Could you check a few things on this model? Use its own coordinates, in mm. Coordinates: 2 decimals unless noted, no trailing zeros. Order: outer loops, then holes, each group sorted by start corner. A loop starts at its lowest first (then second) coordinate and runs counter-clockwise, first axis right, second up. Notation, with made-up numbers: (70, -21.75) -> (102, -21.75) arc R28 ccw to (102, 3.25) -> close; hole circle Ø4 at (6, -34). An arc over 180 degrees is marked (long way). Use a Markdown table: item, result. Add a question column.
1) If we section it at B-B (z = 0): Write out the boundary of the cut face in (x, y), plus the area to 3 significant figures.
2) Thinking about a two-plate mould opening in Z: for faces 1 (the flat face through (6.14, -9, -1)), 2 (the cylindrical face through (-6.106, -11.628, -0.256)), 3 (the cylindrical face through (-16.35, -5.74, -0.07)), which applies, +Z half, -Z half, draft (parallel to the pull), parting line (faces both ways), or undercut?
3) If I drill on L1, parallel to X at y = -9, z = 0; L2, parallel to X at y = -3, z = 0; L3, parallel to Z at x = -14.7, y = -2.5, over which ranges is the centre line in solid material (lowest first)? Write a range as [from, to].
4) If we section it at A-A (y = -2.75): Write out the boundary of the cut face in (x, z), plus the area to 3 significant figures.
5) If we section it at D-D (x = 0): Write out the boundary of the cut face in (y, z).
6) Will these pins go through, and if not, where does the flat tip stop? pin 1 Ø5 at (x, z) = (-15.5, 6) entering from -Y; pin 2 Ø12 at (x, z) = (1, 0.5) entering from +Y; pin 3 Ø4 at (x, y) = (-4, -7) entering from -Z.
7) If we section it at C-C (x = -14.7): Write out the boundary of the cut face in (y, z), plus the area to 3 significant figures.
```python
from build123d import *

# Parameters (mm, degrees)
CORTAR_EXTRUIR5_DEPTH = 50
CROQUIS8_R            = 1.65
CORTAR_EXTRUIR6_DEPTH = 50


with BuildPart() as part:
    # Croquis1 → Revolución4 (revolve)
    with BuildSketch(Plane(origin=(0, 0, 0), x_dir=(1, 0, 0), z_dir=(0, 1, 0))):
        with BuildLine():
            Line((-10.7, 0), (-18.7, 0))
            Line((-18.7, 0), (-18.7, 11.630777084))
            Line((-18.7, 11.630777084), (6.139681858, 11.630777084))
            Line((6.139681858, 11.630777084), (6.139681858, 8.763236085))
            ThreePointArc((6.139681858, 8.763236085), (-4.939403006, 9.491696263), (-10.7, 0))
        make_face()
    revolve(axis=Axis((-10.7, 0, 0), (-1, 0, 0)))

    # Croquis7 → Cortar-Extruir5 (cut)
    with BuildSketch(Plane(origin=(6.139681858, 0, 0), x_dir=(0, 0, -1), z_dir=(1, 0, 0))):
        Polygon((0, 0), (14.104035702, 0), (14.104035702, 12.472423118), (-13.194097915, 12.472423118), (-13.194097915, 0), align=None)
    extrude(amount=-CORTAR_EXTRUIR5_DEPTH, mode=Mode.SUBTRACT)

    # Croquis8 → Cortar-Extruir6 (cut)
    with BuildSketch(Plane(origin=(0, 0, 0), x_dir=(1, 0, 0), z_dir=(0, 1, 0))):
        with Locations((-14.7, 0)):
            Circle(CROQUIS8_R)
    extrude(amount=-CORTAR_EXTRUIR6_DEPTH, mode=Mode.SUBTRACT)


solid = part.part
```
Answer sheet:
| question | item | result |
|---|---|---|
| 1 | outline | (-18.7, -11.63) -> (-16.35, -11.63) -> (-16.35, 0) -> (-18.7, 0) -> close; (-13.05, -11.63) -> (6.14, -11.63) -> (6.14, -8.76) arc R10.7 cw to (-10.7, 0) -> (-13.05, 0) -> close |
| 1 | area | 98.7 mm2 |
| 2 | face 1 | draft |
| 2 | face 2 | parting line |
| 2 | face 3 | undercut |
| 3 | L1 | [-18.7, -16.35], [-13.05, -5.79], [5.79, 6.14] |
| 3 | L2 | [-18.7, -16.35], [-13.05, -10.27] |
| 3 | L3 | [-11.36, -1.65], [1.65, 11.36] |
| 4 | outline | (-18.7, -11.3) -> (6.14, -11.3) -> (6.14, -8.32) arc R10.34 cw (long way) to (6.14, 8.32) -> (6.14, 11.3) -> (-18.7, 11.3) -> close; hole circle Ø3.3 at (-14.7, 0) |
| 4 | area | 266 mm2 |
| 5 | outline | (0, -11.63) -> (0, -10.7) arc R10.7 cw to (0, 10.7) -> (0, 11.63) arc R11.63 ccw to start |
| 6 | pin 1 | y = -11.09 |
| 6 | pin 2 | y = -7.99 |
| 6 | pin 3 | z = -10.5 |
| 7 | outline | (-11.51, -1.65) arc R11.63 ccw to (0, -11.63) -> (0, -1.65) -> close; (-11.51, 1.65) -> (0, 1.65) -> (0, 11.63) arc R11.63 ccw to start |
| 7 | area | 174 mm2 |
